Build history of the part. All positions in model axes, mm. Coordinates: 2 decimals unless noted, no trailing zeros. Order: outer loops, then holes, each group sorted by start corner. A loop starts at its lowest first (then second) coordinate and runs counter-clockwise, first axis right, second up. Notation, with made-up numbers: M 13.5,-17 L 53.5,-17 A21 cw 53.5,-1 Z; hole C -27,-22 d7. An arc over 180 degrees is marked long. Write item = value, one per line. Start each with the question number.
Q1. Pin check, flat tips, straight feed: P1, Ø2.5, axis at x = 34, y = 1.5, coming from the +Z side; P2, Ø1, axis at y = 3, z = 25.5, coming from the -X side; P3, Ø1.5, axis at x = 33, y = 3, coming from the -Z side. Stop position of each tip, or through.
Q2. Drill centre lines: probe 1 along X at (y, z) = (2.25, 10); probe 2 along Z at (x, y) = (-0.5, 2.05); probe 3 along X at (y, z) = (3.9, 32). Where is each one in solid material? Low to high.
Q3. Band-saw the part on A-A on x = 0. Write the cut outline in (y, z).
Q4. Band-saw the part on C-C on y = 2.05. State how many separate pieces and enclosed holes the cut face has, plus the area to 3 significant figures.
Q5. Band-saw the part on B-B on z = 36.5. Write the cut outline in (x, y) (3 decimals), plus the area to 3 significant figures.
Q6. Band-saw the part on D-D on x = -36. Write the cut outline in (y, z), plus the area to 3 significant figures.
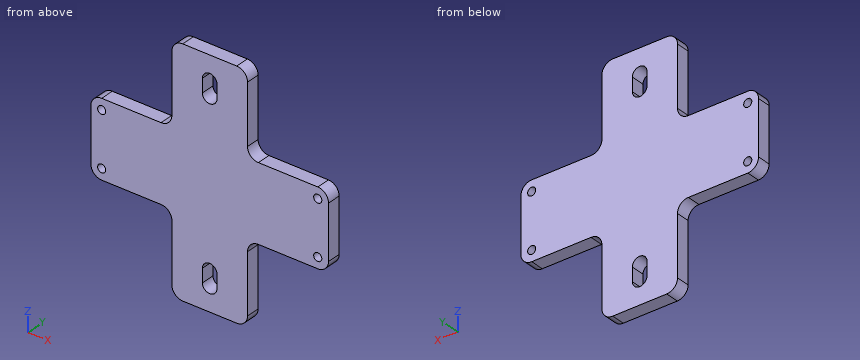
```python
from build123d import *

# Parameters (mm, degrees)
SKETCH_1_R      = 1.5
EXTRUDE_1_DEPTH = 5


with BuildPart() as part:
    # 草图1 → 凸台-拉伸1 (new body)
    with BuildSketch(Plane(origin=(0, 0, 0), x_dir=(1, 0, 0), z_dir=(0, 1, 0))):
        with BuildLine():
            Line((14, -40), (14, -18))
            ThreePointArc((14, -18), (15.171572875, -15.171572875), (18, -14))
            Line((18, -14), (40, -14))
            ThreePointArc((40, -14), (42.828427125, -12.828427125), (44, -10))
            Line((44, -10), (44, 10))
            ThreePointArc((44, 10), (42.828427125, 12.828427125), (40, 14))
            Line((40, 14), (18, 14))
            ThreePointArc((18, 14), (15.171572875, 15.171572875), (14, 18))
            Line((14, 18), (14, 40))
            ThreePointArc((14, 40), (12.828427125, 42.828427125), (10, 44))
            Line((10, 44), (-10, 44))
            ThreePointArc((-10, 44), (-12.828427125, 42.828427125), (-14, 40))
            Line((-14, 40), (-14, 18))
            ThreePointArc((-14, 18), (-15.171572875, 15.171572875), (-18, 14))
            Line((-18, 14), (-40, 14))
            ThreePointArc((-40, 14), (-42.828427125, 12.828427125), (-44, 10))
            Line((-44, 10), (-44, -10))
            ThreePointArc((-44, -10), (-42.828427125, -12.828427125), (-40, -14))
            Line((-40, -14), (-18, -14))
            ThreePointArc((-18, -14), (-15.171572875, -15.171572875), (-14, -18))
            Line((-14, -18), (-14, -40))
            ThreePointArc((-14, -40), (-12.828427125, -42.828427125), (-10, -44))
            Line((-10, -44), (10, -44))
            ThreePointArc((10, -44), (12.828427125, -42.828427125), (14, -40))
        make_face()
        with Locations(Location((40, 10, 0), (0, 0, 270))):
            Circle(SKETCH_1_R, mode=Mode.SUBTRACT)
        with Locations(Location((40, -10, 0), (0, 0, 270))):
            Circle(SKETCH_1_R, mode=Mode.SUBTRACT)
        with Locations(Location((-40, 10, 0), (0, 0, 270))):
            Circle(SKETCH_1_R, mode=Mode.SUBTRACT)
        with Locations(Location((-40, -10, 0), (0, 0, 270))):
            Circle(SKETCH_1_R, mode=Mode.SUBTRACT)
        with BuildLine():
            ThreePointArc((-2.7, 30), (0, 27.3), (2.7, 30))
            Line((2.7, 30), (2.7, 35))
            ThreePointArc((2.7, 35), (0, 37.7), (-2.7, 35))
            Line((-2.7, 35), (-2.7, 30))
        make_face(mode=Mode.SUBTRACT)
        with BuildLine():
            ThreePointArc((2.7, -30), (0, -27.3), (-2.7, -30))
            Line((-2.7, -30), (-2.7, -35))
            ThreePointArc((-2.7, -35), (0, -37.7), (2.7, -35))
            Line((2.7, -35), (2.7, -30))
        make_face(mode=Mode.SUBTRACT)
    extrude(amount=EXTRUDE_1_DEPTH)


solid = part.part
```
Recorded:
q1.P1 = 14
q1.P2 = -14
q1.P3 = -14
q2.probe_1 = -44 to -41.5, -38.5 to 38.5, 41.5 to 44
q2.probe_2 = -44 to -37.65, -27.35 to 27.35, 37.65 to 44
q2.probe_3 = -14 to -2.7, 2.7 to 14
q3.outline = M 0,-44 L 5,-44 L 5,-37.7 L 0,-37.7 Z; M 0,-27.3 L 5,-27.3 L 5,27.3 L 0,27.3 Z; M 0,37.7 L 5,37.7 L 5,44 L 0,44 Z
q4.separate_pieces = 1
q4.enclosed_holes = 6
q4.area = 4,000 mm2
q5.outline = M -14,0 L -2.245,0 L -2.245,5 L -14,5 Z; M 2.245,0 L 14,0 L 14,5 L 2.245,5 Z
q5.area = 118 mm2
q6.outline = M 0,-14 L 5,-14 L 5,14 L 0,14 Z
q6.area = 140 mm2
